For this review, take the finished solid that the model builds, in its own axes (mm). Face numbers are marked on the shaded views. A direction names the side the tool comes from. Give positions to 0.01 mm unless a question says otherwise; leave off trailing zeros. Loops run counter-clockwise (first coordinate to the right, second up) from the corner with the lowest first, then second, coordinate; pieces in that order, holes last. Notation, with made-up numbers: M -30.5,17 L 12.5,17 A17 cw 12.5,38 Z; hole C -36,-31.5 d3. An arc over 180 degrees is marked long. Use CSV: the item, a comma, the result in double quotes. Start each with the question number.
1. Tool access review of the marked faces 1, 2 and 3: name each direction out of +Z, -Z, +X, -X, +Y, -Y from which nothing blocks a thin tool from reaching the whole face with its end or side.
2. Insertion check: P1, Ø9, axis at x = 422.5, y = -92, coming from the +Z side; P2, Ø12.5, axis at x = 422.5, y = 92, coming from the +Z side; P3, Ø14.5, axis at x = 25, y = 92, coming from the -Z side; P4, Ø8, axis at x = 254.5, z = -7, coming from the -Y side. Each pin has a flat end and moves straight along its axis. Give the tip position at first contact, or say it passes through.
3. Take a section at B-B, the plane y = -92. State how many separate pieces and enclosed holes the cut face has, and give its area (3 significant figures).
4. Take a section at A-A, the plane x = 157.5. Write out the cut boundary in (y, z), and give its area (3 significant figures).
5. To check wall thickness, follow line 1 (Y direction, x = 422.5, z = 14); line 2 (Y direction, x = 28, z = 31); line 3 (Z direction, x = 143.5, y = -70). State the ranges of each line that lie inside material, in increasing order. Write a range as [from, to].
6. Take a section at C-C, the plane x = 485.5. Write out the cut boundary in (y, z).
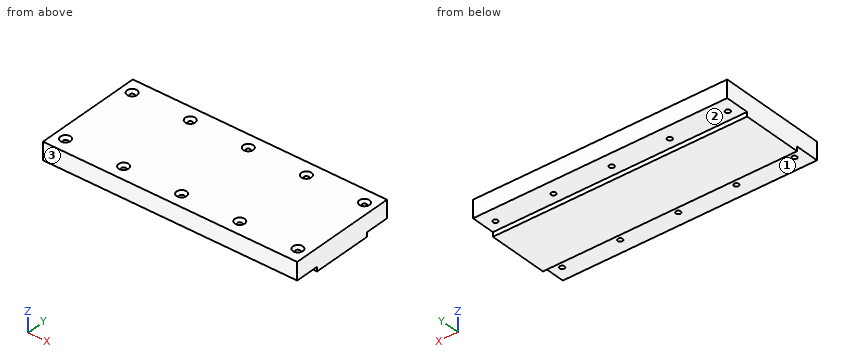
from build123d import *

# Parameters (mm, degrees)
BOSS_EXTRUDE1_DEPTH = 580
SKETCH2_R           = 5.5
CUT_EXTRUDE1_DEPTH  = 596.210886997
CHAMFER1_SIZE       = 6


with BuildPart() as part:
    # Sketch1 → Boss-Extrude1 (new body)
    with BuildSketch(Plane(origin=(0, 0, 0), x_dir=(0, 0, -1), z_dir=(1, 0, 0))):
        Polygon((0, -124), (-40, -124), (-40, 124), (0, 124), (0, 69), (10, 69), (10, -69), (0, -69), align=None)
    extrude(amount=BOSS_EXTRUDE1_DEPTH)

    # Sketch2 → Cut-Extrude1 (cut, through all)
    with BuildSketch(Plane.XY.offset(40)):
        with Locations((25, 92)):
            Circle(SKETCH2_R)
        with Locations((157.5, 92)):
            Circle(SKETCH2_R)
        with Locations(Location((422.5, 92, 0), (0, 0, 270))):
            Circle(SKETCH2_R)
        with Locations(Location((555, 92, 0), (0, 0, 270))):
            Circle(SKETCH2_R)
        with Locations((290, 92)):
            Circle(SKETCH2_R)
        with Locations((555, -92)):
            Circle(SKETCH2_R)
        with Locations((422.5, -92)):
            Circle(SKETCH2_R)
        with Locations(Location((290, -92, 0), (0, 0, 270))):
            Circle(SKETCH2_R)
        with Locations(Location((157.5, -92, 0), (0, 0, 270))):
            Circle(SKETCH2_R)
        with Locations(Location((25, -92, 0), (0, 0, 270))):
            Circle(SKETCH2_R)
    extrude(amount=-CUT_EXTRUDE1_DEPTH, mode=Mode.SUBTRACT)

    # Chamfer1
    chamfer1_edges = [part.edges().sort_by_distance(p)[0] for p in [
        (25, -86.5, 40),
        (157.5, -86.5, 40),
        (290, -86.5, 40),
        (417, -92, 40),
        (549.5, -92, 40),
        (152, 92, 40),
        (422.5, 97.5, 40),
        (555, 97.5, 40),
        (284.5, 92, 40),
        (19.5, 92, 40),
    ]]
    chamfer(chamfer1_edges, length=CHAMFER1_SIZE)


solid = part.part
Result set:
1,face 1,"-Z, +X, -X, -Y"
1,face 2,"-Z, +X, -X, +Y"
1,face 3,"+Z, -Z, +X, -X, -Y"
2,P1,"through"
2,P2,"z = 34.75"
2,P3,"z = 0"
2,P4,"y = -69"
3,separate pieces,"6"
3,enclosed holes,"0"
3,area,"20,800 mm2"
4,outline,"M -124,0 L -97.5,0 L -97.5,34 L -103.5,40 L -124,40 Z; M -86.5,0 L -69,0 L -69,-10 L 69,-10 L 69,0 L 86.5,0 L 86.5,34 L 80.5,40 L -80.5,40 L -86.5,34 Z; M 97.5,0 L 124,0 L 124,40 L 103.5,40 L 97.5,34 Z"
4,area,"10,300 mm2"
5,line 1,"[-124, -97.5], [-86.5, 86.5], [97.5, 124]"
5,line 2,"[-124, -96.61], [-87.39, 87.39], [96.61, 124]"
5,line 3,"[0, 40]"
6,outline,"M -124,0 L -69,0 L -69,-10 L 69,-10 L 69,0 L 124,0 L 124,40 L -124,40 Z"
